Work out the finished part from the listing and answer in its coordinate system (mm). Face numbers are marked on the shaded views. A direction names the side the tool comes from. Give positions to 0.01 mm unless a question says otherwise; leave off trailing zeros. Loops run counter-clockwise (first coordinate to the right, second up) from the corner with the lowest first, then second, coordinate; pieces in that order, holes last. Notation, with made-up numbers: (4.25, 21.25) - (51.25, 21.25) arc R11 ccw to (51.25, 30.25) - close; hole circle Ø9 at (43, 62). An arc over 180 degrees is marked (long way). One line per question, with ' | ' between items.
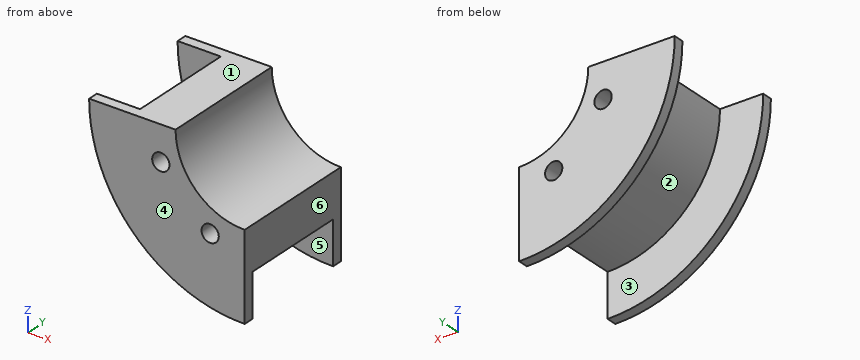
from build123d import *

# Parameters (mm, degrees)
REVOLVE_1_ANGLE     = 90
SKETCH_2_R          = 1
CUT_EXTRUDE_1_DEPTH = 27.795522014


with BuildPart() as part:
    # 草图1 → 旋转1 (revolve)
    with BuildSketch(Plane.XY):
        Polygon((-5, 7.5), (5, 7.5), (5, -7.5), (-5, -7.5), (-5, -6.3), (0, -6.3), (0, 6.3), (-5, 6.3), align=None)
    revolve(axis=Axis((13, 23.403849413, 0), (0, -1, 0)), revolution_arc=REVOLVE_1_ANGLE)

    # 草图2 → 切除-拉伸1 (cut, through all)
    with BuildSketch(Plane.XZ.offset(7.5)):
        with Locations((3.291756081, -4)):
            Circle(SKETCH_2_R)
        with Locations((9, -9.708243919)):
            Circle(SKETCH_2_R)
    extrude(amount=-CUT_EXTRUDE_1_DEPTH, mode=Mode.SUBTRACT)


solid = part.part
1. Flat-ended cylindrical pins translate along their axes: pin 1 (8 mm diameter, centred on x = -3, y = 0.5, fed in from +Z); pin 2 (5 mm diameter, centred on x = 7, y = 3, fed in from -Z); pin 3 (1 mm diameter, centred on y = -0.5, z = -14, fed in from +X); pin 4 (4 mm diameter, centred on y = -3, z = -6.5, fed in from -X). Find the tip coordinate at first contact, or state that the pin passes through.
Evaluation:
pin 1: z = 0 | pin 2: z = -12.52 | pin 3: through | pin 4: x = 0.8
2. Which of the six approach directions +Z, -Z, +X, -X, +Y, -Y give full straight-line access (tool end or side, diameter ignored) to the marked faces 5 and 6?
Evaluation:
face 5: -Z, -X | face 6: +Z, -Z, +X, +Y, -Y
3. Find section B-B on z = -4.25. Write down the section's boundary in (x, y).
Evaluation:
outline: (-4.49, -7.5) - (2.32, -7.5) - (2.32, 7.5) - (-4.49, 7.5) - (-4.49, 6.3) - (0.71, 6.3) - (0.71, -6.3) - (-4.49, -6.3) - close; (4.26, -7.5) - (6.22, -7.5) - (6.22, 7.5) - (4.26, 7.5) - close
4. Consider L1, parallel to Y at x = 9, z = -13.5; L2, parallel to Z at x = 9, y = -2; L3, parallel to X at y = 6.25, z = -10.5. Determine where each line is inside the solid, lowest interval first.
Evaluation:
L1: -7.5 to -6.3, 6.3 to 7.5 | L2: -12.37 to -10.71, -8.71 to -6.93 | L3: 5.34 to 8.39, 9.61 to 13
5. Find section D-D on x = 11.25. Write down the section's boundary in (y, z).
Evaluation:
outline: (-7.5, -17.91) - (-6.3, -17.91) - (-6.3, -12.88) - (6.3, -12.88) - (6.3, -17.91) - (7.5, -17.91) - (7.5, -7.81) - (-7.5, -7.81) - close
6. Find section C-C on z = -0.75. Write down the section's boundary in (x, y).
Evaluation:
outline: (-4.98, -7.5) - (5.04, -7.5) - (5.04, 7.5) - (-4.98, 7.5) - (-4.98, 6.3) - (0.02, 6.3) - (0.02, -6.3) - (-4.98, -6.3) - close
7. Determine the mould class of the marked faces 1, 2, 3 and 4 for opening direction Y: +Y half, -Y half, draft (parallel to the pull), parting line (faces both ways), or undercut.
Evaluation:
face 1: draft | face 2: undercut | face 3: undercut | face 4: -Y half
8. Find section A-A on x = -1.5. Write down the section's boundary in (y, z).
Evaluation:
outline: (-7.5, -10.67) - (-6.3, -10.67) - (-6.3, 0) - (-7.5, 0) - close; (6.3, -10.67) - (7.5, -10.67) - (7.5, 0) - (6.3, 0) - close
